from build123d import *

# Parameters (mm, degrees)
SKETCH_W      = 80
SKETCH_H      = 80
PAD_DEPTH     = 2.5
SKETCH001_R   = 38.5
SKETCH001_R_2 = 1.75
POCKET_DEPTH  = 5
PAD001_DEPTH  = 2.5
SKETCH003_R   = 32.5
SKETCH003_R_2 = 31.5
PAD002_DEPTH  = 2.5
SKETCH004_R   = 25
SKETCH004_R_2 = 24
PAD003_DEPTH  = 2.5
SKETCH005_R   = 17.5
SKETCH005_R_2 = 16.5
PAD004_DEPTH  = 2.5
FILLET_R      = 4
FILLET001_R   = 5


with BuildPart() as part:
    # Sketch → Pad (new body)
    with BuildSketch(Plane.XY):
        Rectangle(SKETCH_W, SKETCH_H)
    extrude(amount=PAD_DEPTH)

    # Sketch001 (on Face6 of Pad) → Pocket (cut)
    with BuildSketch(Plane.XY.offset(2.5)):
        Circle(SKETCH001_R)
        with Locations((35.75, 35.75)):
            Circle(SKETCH001_R_2)
        with Locations((-35.75, 35.75)):
            Circle(SKETCH001_R_2)
        with Locations((-35.75, -35.75)):
            Circle(SKETCH001_R_2)
        with Locations((35.75, -35.75)):
            Circle(SKETCH001_R_2)
    extrude(amount=-POCKET_DEPTH, mode=Mode.SUBTRACT)

    # Sketch002 (on Face4 of Pocket) → Pad001 (join)
    with BuildSketch(Plane(origin=(0, 0, 0), x_dir=(1, 0, 0), z_dir=(0, 0, -1))):
        Polygon((1.5, 39.224094), (-1.5, 39.224094), (-1.5, 1.5), (-39.182049, 1.5), (-39.182049, -1.5), (-1.5, -1.5), (-1.5, -39.571514), (1.5, -39.571514), (1.5, -1.5), (38.958385, -1.5), (38.958385, 1.5), (1.5, 1.5), align=None)
    extrude(amount=-PAD001_DEPTH)

    # Sketch003 (on Face23 of Pad001) → Pad002 (join)
    with BuildSketch(Plane(origin=(0, 0, 0), x_dir=(1, 0, 0), z_dir=(0, 0, -1))):
        Circle(SKETCH003_R)
        Circle(SKETCH003_R_2, mode=Mode.SUBTRACT)
    extrude(amount=-PAD002_DEPTH)

    # Sketch004 (on Face53 of Pad002) → Pad003 (join)
    with BuildSketch(Plane(origin=(0, 0, 0), x_dir=(1, 0, 0), z_dir=(0, 0, -1))):
        Circle(SKETCH004_R)
        Circle(SKETCH004_R_2, mode=Mode.SUBTRACT)
    extrude(amount=-PAD003_DEPTH)

    # Sketch005 (on Face89 of Pad003) → Pad004 (join)
    with BuildSketch(Plane(origin=(0, 0, 0), x_dir=(1, 0, 0), z_dir=(0, 0, -1))):
        Circle(SKETCH005_R)
        Circle(SKETCH005_R_2, mode=Mode.SUBTRACT)
    extrude(amount=-PAD004_DEPTH)

    # Fillet
    fillet_edges = [part.edges().sort_by_distance(p)[0] for p in [
        (-40, 40, 1.25),
        (40, 40, 1.25),
        (40, -40, 1.25),
        (-40, -40, 1.25),
    ]]
    fillet(fillet_edges, radius=FILLET_R)

    # Fillet001
    fillet001_edges = [part.edges().sort_by_distance(p)[0] for p in [
        (-1.5, 1.5, 1.25),
        (-1.5, -1.5, 1.25),
        (1.5, -1.5, 1.25),
        (1.5, 1.5, 1.25),
    ]]
    fillet(fillet001_edges, radius=FILLET001_R)


solid = part.part
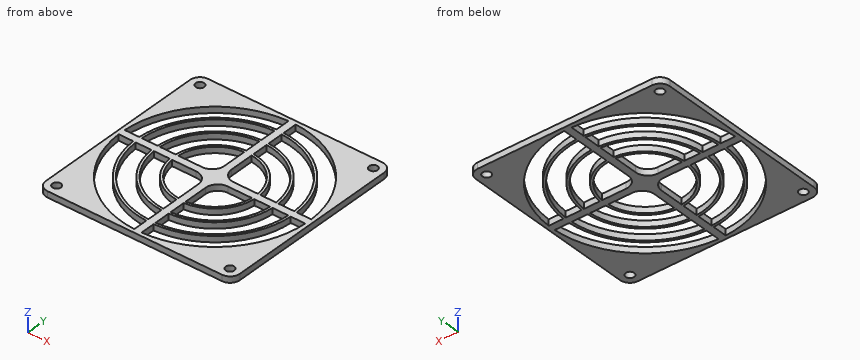
CAD build for the part. Positions are in the model's coordinates, mm. Give positions to 0.01 mm unless a question says otherwise; leave off trailing zeros. Write each loop counter-clockwise with the first axis right and the second up, starting at its lowest first coordinate (ties: lowest second). Pieces come first, ordered by that corner, then holes. Notation, with made-up numbers: (-8, 25.5) - (0, 25.5) arc R23 ccw to (0, 51.5) - close; hole circle Ø8 at (5, 65.5). An arc over 180 degrees is marked (long way). Put each result on its own line as item: value.
(1) Saw through at B-B (z = 1.85). Count the separate pieces of the cut face and the enclosed holes in it, then the cut area to 3 significant figures.
Working result:
separate pieces: 1
enclosed holes: 20
area: 2,590 mm^2
(2) Wall check: L1, parallel to Y at x = -35.75, z = 1.9; L2, parallel to Y at x = 35.5, z = 1.55. Give the ranges that are in metal, low to high.
Working result:
L1: -40 to -37.5, -34 to -14.29, -1.5 to 1.5, 14.29 to 34, 37.5 to 40
L2: -40 to -37.48, -34.02 to -14.9, -1.5 to 1.5, 14.9 to 34.02, 37.48 to 40
(3) Drop flat-ended pins along their axis: pin 1 Ø2 at (x, y) = (35.75, -35.75) entering from -Z; pin 2 Ø8 at (x, y) = (12, -26) entering from +Z. Give the stop position or say it passes through.
Working result:
pin 1: through
pin 2: z = 2.5
(4) Saw through at A-A (x = -29.5). List the corners of the cut face in (y, z).
Working result:
outline: (-40, 0) - (-24.74, 0) - (-24.74, 2.5) - (-40, 2.5) - close; (-13.64, 0) - (-11.05, 0) - (-11.05, 2.5) - (-13.64, 2.5) - close; (-1.5, 0) - (1.5, 0) - (1.5, 2.5) - (-1.5, 2.5) - close; (11.05, 0) - (13.64, 0) - (13.64, 2.5) - (11.05, 2.5) - close; (24.74, 0) - (40, 0) - (40, 2.5) - (24.74, 2.5) - close
